Here's the drawing with two shaded views (mm, measured from the low corner). I have some questions. Coordinates: 2 decimals unless noted, no trailing zeros. Loops run counter-clockwise (first coordinate to the right, second up) from the corner with the lowest first, then second, coordinate; pieces in that order, holes last. Notation, with made-up numbers: (73, -22.5) -> (128, -22.5) arc R12 ccw to (128, -5.5) -> close; hole circle Ø10 at (-1.75, 57.25). An arc over 180 degrees is marked (long way). Answer as a JSON object with one key per item and string values. Group by question number.
Q1. I need wall thicknesses on line 1 (Z direction, x = 151, y = 5.5) (1 decimal); line 2 (X direction, y = 4, z = 123) (1 decimal); line 3 (X direction, y = 5.75, z = 14). Which ranges of each line are inside material? Lowest first, please.
Q2. I'm going to push flat-ended pins straight in: pin 1 (1.5 mm diameter, centred on y = 1, z = 107.5, fed in from -X); pin 2 (1.5 mm diameter, centred on y = 4, z = 23, fed in from +X); pin 3 (1 mm diameter, centred on x = 161, y = 4, fed in from -Z). Where does each tip first touch, or does it pass through?
Q3. I want a section at B-B on z = 16.5. Write out the boundary of the cut face in (x, y), then the cut area to 3 significant figures.
Q4. I want a section at A-A on x = 101. Write out the boundary of the cut face in (y, z), then the cut area to 3 significant figures.
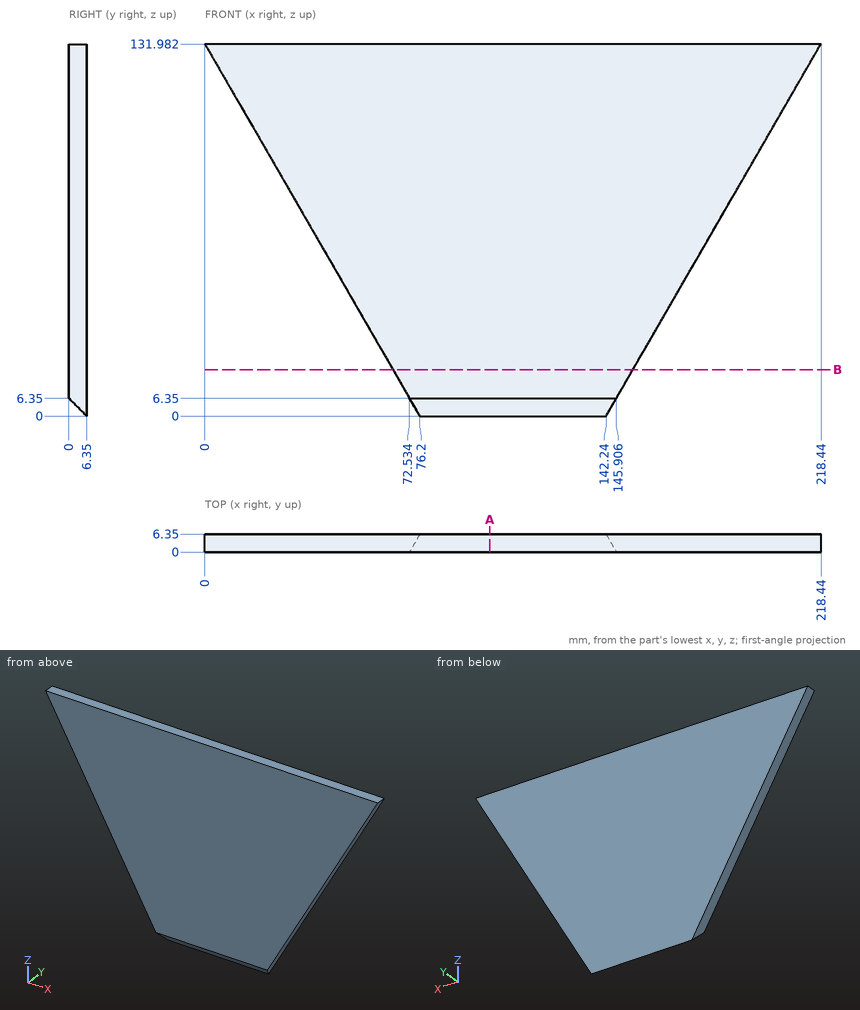
Result set:
{
 "1": {"line 1": "z = 15.2 to 132", "line 2": "x = 5.2 to 213.3", "line 3": "x = 68.12 to 150.32"},
 "2": {"pin 1": "stops at x = 13.7", "pin 2": "stops at x = 155.95", "pin 3": "stops at z = 31.63"},
 "3": {"outline": "(66.67, 0) -> (151.77, 0) -> (151.77, 6.35) -> (66.67, 6.35) -> close", "area": "540 mm²"},
 "4": {"outline": "(0, 6.35) -> (6.35, 0) -> (6.35, 131.98) -> (0, 131.98) -> close", "area": "818 mm²"}
}
